Part print with two shaded views. Sizes in mm from the minimum x, y, z corner. Coordinates: 2 decimals unless noted, no trailing zeros. Loops run counter-clockwise (first coordinate to the right, second up) from the corner with the lowest first, then second, coordinate; pieces in that order, holes last.
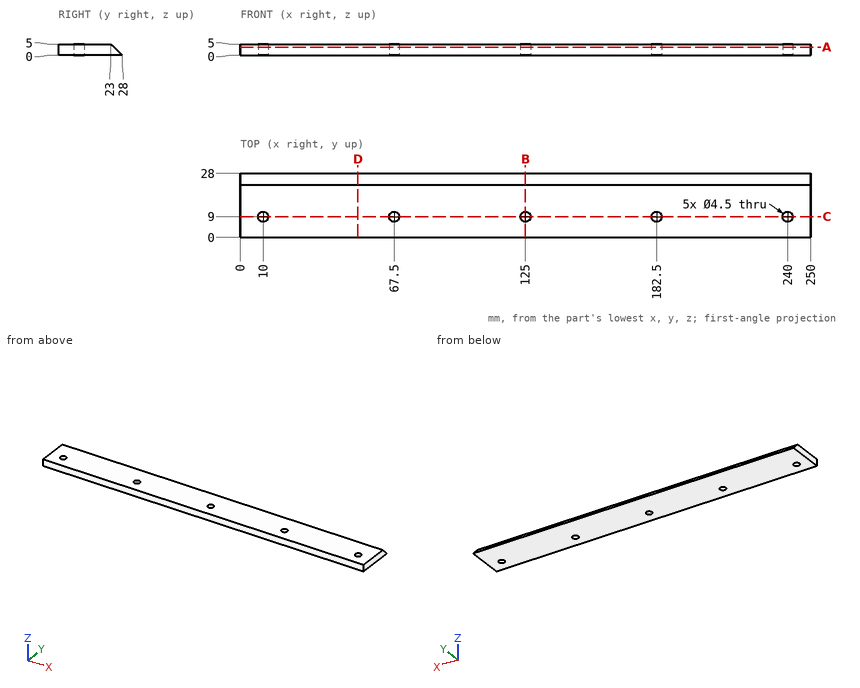
Q1. Drill centre lines: line 1 (X direction, y = 9.25, z = 3.55); line 2 (X direction, y = 7.25, z = 2.8); line 3 (Y direction, x = 182.5, z = 2.35). Where is each one in solid material? Low to high.
Answers:
line 1: x = 0 to 7.76, 12.24 to 65.26, 69.74 to 122.76, 127.24 to 180.26, 184.74 to 237.76, 242.24 to 250
line 2: x = 0 to 8.59, 11.41 to 66.09, 68.91 to 123.59, 126.41 to 181.09, 183.91 to 238.59, 241.41 to 250
line 3: y = 0 to 6.75, 11.25 to 25.65
Q2. Slice it at D-D (x = 51.5). List the corners of the cut face in (y, z), and give its area (4 significant figures).
Answers:
outline: (0, 0) - (28, 0) - (23, 5) - (0, 5) - close
area: 127.5 mm2
Q3. Flat gauge pin, fed straight in: P1, Ø5, axis at x = 10, y = 9, coming from the -Z side. Where does the tip first touch, or does it go through?
Answers:
P1: stops at z = 0
Q4. Slice it at A-A (z = 3.65). List the corners of the cut face in (x, y).
Answers:
outline: (0, 0) - (250, 0) - (250, 24.35) - (0, 24.35) - close; hole circle Ø4.5 at (10, 9); hole circle Ø4.5 at (67.5, 9); hole circle Ø4.5 at (125, 9); hole circle Ø4.5 at (182.5, 9); hole circle Ø4.5 at (240, 9)
Q5. Slice it at C-C (y = 9). List the corners of the cut face in (x, z).
Answers:
outline: (0, 0) - (7.75, 0) - (7.75, 5) - (0, 5) - close; (12.25, 0) - (65.25, 0) - (65.25, 5) - (12.25, 5) - close; (69.75, 0) - (122.75, 0) - (122.75, 5) - (69.75, 5) - close; (127.25, 0) - (180.25, 0) - (180.25, 5) - (127.25, 5) - close; (184.75, 0) - (237.75, 0) - (237.75, 5) - (184.75, 5) - close; (242.25, 0) - (250, 0) - (250, 5) - (242.25, 5) - close
Q6. Slice it at B-B (x = 125). List the corners of the cut face in (y, z).
Answers:
outline: (0, 0) - (6.75, 0) - (6.75, 5) - (0, 5) - close; (11.25, 0) - (28, 0) - (23, 5) - (11.25, 5) - close
